from build123d import *

# Parameters (mm, degrees)
SKETCH1_W                           = 32
SKETCH1_H                           = 12
BOSS_EXTRUDE1_DEPTH                 = 10
TAP_DRILL_FOR_M3X0_5_TAP1_D         = 2.5
TAP_START                           = -12
TAP_DRILL_FOR_M3X0_5_TAP2_OUTLINE_R = 1.25
TAP_DRILL_FOR_M3X0_5_TAP2_DEPTH     = 12


# Read off the part's stored shape, not the designer's step: Tap Drill for M3x0.5 Tap2
with BuildPart() as part:
    # Sketch1 → Boss-Extrude1 (new body)
    with BuildSketch(Plane(origin=(0, 0, 0), x_dir=(1, 0, 0), z_dir=(0, 1, 0))):
        with Locations((16, 6)):
            Rectangle(SKETCH1_W, SKETCH1_H)
    extrude(amount=BOSS_EXTRUDE1_DEPTH)

    # Tap Drill for M3x0.5 Tap1 (through all)
    with Locations(Plane(origin=(0, 10, 0), x_dir=(1, 0, 0), z_dir=(0, 1, 0))):
        with Locations((6, 6)):
            Hole(TAP_DRILL_FOR_M3X0_5_TAP1_D / 2)

    # Tap Drill for M3x0.5 Tap2 outline → Tap Drill for M3x0.5 Tap2 (cut)
    with BuildSketch(Plane.XY.offset(TAP_START)):
        with Locations((16, 5)):
            Circle(TAP_DRILL_FOR_M3X0_5_TAP2_OUTLINE_R)
        with Locations((28, 5)):
            Circle(TAP_DRILL_FOR_M3X0_5_TAP2_OUTLINE_R)
    extrude(amount=TAP_DRILL_FOR_M3X0_5_TAP2_DEPTH, mode=Mode.SUBTRACT)


solid = part.part
CAD build for the part. Positions are in the model's coordinates, mm. Coordinates: 2 decimals unless noted, no trailing zeros. Loops run counter-clockwise (first coordinate to the right, second up) from the corner with the lowest first, then second, coordinate; pieces in that order, holes last. Notation, with made-up numbers: (1.5, 55.5) - (24.5, 55.5) arc R14 cw to (24.5, 74.5) - close; hole circle Ø10 at (-33, 58). An arc over 180 degrees is marked (long way). Use one line per item in the form item = value. Start each with the question number.
1) Band-saw the part on C-C (x = 6). Give the cut face in (y, z), and give its area (3 significant figures).
2) Band-saw the part on A-A (y = 5.75). Give the cut face in (x, z).
3) Band-saw the part on B-B (z = -6.75). Give the cut face in (x, y), and give its area (3 significant figures).
4) Band-saw the part on D-D (z = -11). Give the cut face in (x, y).
5) Drill centre lines: L1, parallel to Y at x = 28, z = -8.75; L2, parallel to Z at x = 6, y = 2.5; L3, parallel to X at y = 0.75, z = -7. Where is each one in solid material? Low to high. Write a range as from..to.
6) Two-plate mould, pull along X, no slides. Class faces 1 (the face through (32, 5, -6)), 2 (the face through (15.73, 3.78, -6.08)), 3 (the face through (16, 10, -6)): +X half, -X half, draft (parallel to the pull), parting line (faces both ways), or undercut.
Check values:
q1.outline = (0, -12) - (10, -12) - (10, -7.25) - (0, -7.25) - close; (0, -4.75) - (10, -4.75) - (10, 0) - (0, 0) - close
q1.area = 95.0 mm2
q2.outline = (0, -12) - (15, -12) - (15, 0) - (0, 0) - close; (17, -12) - (27, -12) - (27, 0) - (17, 0) - close; (29, -12) - (32, -12) - (32, 0) - (29, 0) - close; hole circle Ø2.5 at (6, -6)
q3.outline = (0, 0) - (5, 0) - (5, 10) - (0, 10) - close; (7, 0) - (32, 0) - (32, 10) - (7, 10) - close; hole circle Ø2.5 at (16, 5); hole circle Ø2.5 at (28, 5)
q3.area = 290 mm2
q4.outline = (0, 0) - (32, 0) - (32, 10) - (0, 10) - close; hole circle Ø2.5 at (16, 5); hole circle Ø2.5 at (28, 5)
q5.L1 = 0..3.75, 6.25..10
q5.L2 = -12..-7.25, -4.75..0
q5.L3 = 0..5.25, 6.75..32
q6.face_1 = +X half
q6.face_2 = undercut
q6.face_3 = draft
